Verification items for the finished model (mm, model axes). Face numbers are marked on the shaded views. A direction names the side the tool comes from. Give positions to 0.01 mm unless a question says otherwise; leave off trailing zeros. Order: outer loops, then holes, each group sorted by start corner. A loop starts at its lowest first (then second) coordinate and runs counter-clockwise, first axis right, second up. Notation, with made-up numbers: (-29.75, 45.5) - (-5.75, 45.5) arc R27 cw to (-5.75, 71.5) - close; hole circle Ø10 at (82, 2.5). An arc over 180 degrees is marked (long way). Answer as a JSON object with one key per item and string values. Group by question number.
(1) Access from +Z, -Z, +X, -X, +Y, -Y to the whole of each face (thin tool, end or side, straight path). Record for the marked faces 5, 6 and 7.
(2) Mould release check, pull along Z, two halves, no side actions. Record for the marked faces 1, 2, 3 and 4: +Z half, -Z half, draft (parallel to the pull), parting line (faces both ways), or undercut.
(3) Section check D-D (x = -7.5). Record the boundary of the cut face in (y, z), then the cut area to 3 significant figures.
(4) Thickness scan on line 1 (Y direction, x = -18, z = 0); line 2 (Y direction, x = -12.5, z = -0.25); line 3 (Z direction, x = -10.75, y = 5.25). Record the ranges inside material, lowest first.
(5) Section check B-B (x = -16.25). Record the boundary of the cut face in (y, z).
(6) Depth check by flat-ended pin: pin 1 Ø1 at (x, y) = (-4, 4.5) entering from -Z; pin 2 Ø4 at (x, z) = (-10.5, 9) entering from +Y; pin 3 Ø1 at (x, y) = (-18.5, -6) entering from +Z; pin 4 Ø1.1 at (y, z) = (8, 0) entering from -X. Enter the tip coordinate at first touch or a pass-through.
(7) Section check A-A (z = 0). Record the boundary of the cut face in (x, y).
(8) Section check C-C (y = 0). Record the boundary of the cut face in (x, z).
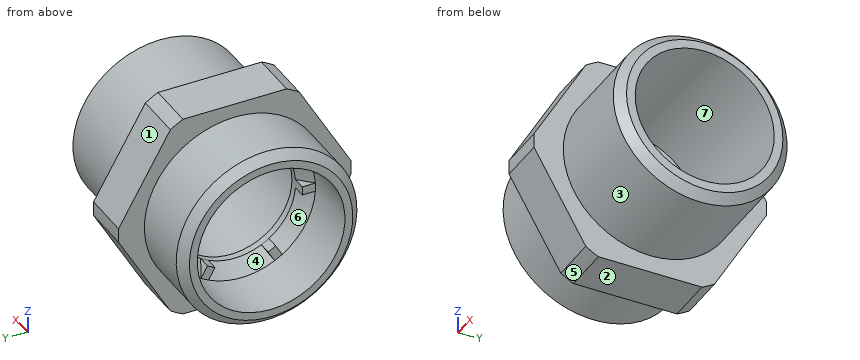
```python
from build123d import *

# Parameters (mm, degrees)
SKETCH_2_R               = 10
EXTRUDE_1_DEPTH          = 12
SKETCH_3_R               = 10
EXTRUDE_2_DEPTH          = 5.5
SKETCH_4_R               = 10.4
EXTRUDE_3_DEPTH          = 8
SKETCH_6_R               = 13.856406461
SKETCH_6_R_2             = 13.4
CUT_EXTRUDE_1_DEPTH      = 26.342651795
CHAMFER_1_SIZE           = 1
EXTRUDE_4_REACH          = 26.545
SKETCH_7_W               = 1
SKETCH_7_H               = 8.5
SKETCH_8_R               = 7
CUT_EXTRUDE_2_DEPTH      = 32.205928924
SKETCH_9_R               = 8.5
CUT_EXTRUDE_3_DEPTH      = 6.5
PATTERN_CIRCULAR_1_COUNT = 6


with BuildPart() as part:
    # Эскиз2 → Вытянуть1 (new body)
    with BuildSketch(Plane(origin=(0, 0, 0), x_dir=(0, 0, -1), z_dir=(1, 0, 0))):
        Circle(SKETCH_2_R)
    extrude(amount=-EXTRUDE_1_DEPTH)

    # Эскиз3 → Вытянуть2 (add)
    # profile 1 of 2: a face of its own
    with BuildSketch(Plane.ZY.offset(12)):
        Polygon((12, -6.92820323), (12, 6.92820323), (0, 13.856406461), (-12, 6.92820323), (-12, -6.92820323), (0, -13.856406461), align=None)
        with Locations(Location((0, 0, 0), (0, 0, 180))):
            Circle(SKETCH_3_R, mode=Mode.SUBTRACT)
    # profile 2 of 2: a face of its own
    with BuildSketch(Plane.ZY.offset(12)):
        with Locations(Location((0, 0, 0), (0, 0, 180))):
            Circle(SKETCH_3_R)
    extrude(amount=EXTRUDE_2_DEPTH)

    # Эскиз4 → Вытянуть3 (add)
    with BuildSketch(Plane.ZY.offset(17.5)):
        Circle(SKETCH_4_R)
    extrude(amount=EXTRUDE_3_DEPTH)

    # Эскиз5 → Вырез-Повернуть1 (revolve, cut)
    with BuildSketch(Plane.XY, mode=Mode.PRIVATE) as cut_revolve_1_sk:
        Polygon((0, 0), (0, 8), (-16.7, 8), (-16.7, 7), (-17.5, 7), (-19, 8.5), (-25.5, 8.5), (-25.5, 0), align=None)
    revolve(cut_revolve_1_sk.sketch.rotate(Axis((-25.5, 0, 0), (1, 0, 0)), 90), axis=Axis((-25.5, 0, 0), (1, 0, 0)), mode=Mode.SUBTRACT)

    # Эскиз6 → Вырез-Вытянуть1 (cut, through all)
    with BuildSketch(Plane.ZY.offset(17.5)):
        Circle(SKETCH_6_R)
        Circle(SKETCH_6_R_2, mode=Mode.SUBTRACT)
    extrude(amount=-CUT_EXTRUDE_1_DEPTH, mode=Mode.SUBTRACT)

    # Фаска1
    chamfer_1_edges = [part.edges().sort_by_distance(p)[0] for p in [
        (0, 0, 10),
        (-25.5, 0, -10.4),
    ]]
    chamfer(chamfer_1_edges, length=CHAMFER_1_SIZE)

    # Вытянуть4: up to this face of the body (flat: up to its plane)
    extrude_4_end = Plane(part.part.faces().sort_by_distance((-25.5, 0, -9.13412785))[0])
    # Эскиз7 → Вытянуть4 (add, up to the picked face)
    with BuildSketch(Plane(origin=(-16.7, 0, 0), x_dir=(0, 0, -1), z_dir=(1, 0, 0)), mode=Mode.PRIVATE) as extrude_4_sk1:
        with Locations((0, 4.25)):
            Rectangle(SKETCH_7_W, SKETCH_7_H)
    extrude_4_tool1 = split(extrude(extrude_4_sk1.sketch, amount=-EXTRUDE_4_REACH, mode=Mode.PRIVATE), bisect_by=extrude_4_end, keep=Keep.BOTH, mode=Mode.PRIVATE)
    add(extrude_4_tool1.solids().sort_by(Axis((-16.7, 4.25, 0), (-1, 0, 0)))[0])

    # Эскиз8 → Вырез-Вытянуть2 (cut, through all)
    with BuildSketch(Plane.ZY.offset(25.5)):
        Circle(SKETCH_8_R)
    extrude(amount=-CUT_EXTRUDE_2_DEPTH, mode=Mode.SUBTRACT)

    # Эскиз9 → Вырез-Вытянуть3 (cut)
    with BuildSketch(Plane.ZY.offset(25.5)):
        Circle(SKETCH_9_R)
    extrude(amount=-CUT_EXTRUDE_3_DEPTH, mode=Mode.SUBTRACT)

    # Круговой массив1: part ×6 about axis
    pattern_circular_1_axis = Axis((0, 0, 0), (1, 0, 0))


with BuildPart() as part_1:
    add(part.part)
    for i in range(1, PATTERN_CIRCULAR_1_COUNT):
        add(part.part.rotate(pattern_circular_1_axis, i * 360 / PATTERN_CIRCULAR_1_COUNT))


solid = part_1.part
```
Solutions:
{
 "1": {"face 5": "-Z, +X, -X, -Y", "face 6": "-X", "face 7": "+X"},
 "2": {"face 1": "+Z half", "face 2": "-Z half", "face 3": "parting line", "face 4": "undercut"},
 "3": {"outline": "circle Ø20 at (0, 0); hole circle Ø16 at (0, 0)", "area": "113 mm2"},
 "4": {"line 1": "y = -10.4 to -7, 7 to 10.4", "line 2": "y = -13.4 to -8, 8 to 13.4", "line 3": "z = -8.51 to -6.04, 6.04 to 8.51"},
 "5": {"outline": "(-13.37, -0.84) - (-7.41, -11.16) arc R13.4 ccw to (-5.96, -12) - (5.96, -12) arc R13.4 ccw to (7.41, -11.16) - (13.37, -0.84) arc R13.4 ccw to (13.37, 0.84) - (7.41, 11.16) arc R13.4 ccw to (5.96, 12) - (-5.96, 12) arc R13.4 ccw to (-7.41, 11.16) - (-13.37, 0.84) arc R13.4 ccw to start; hole circle Ø16 at (0, 0)"},
 "6": {"pin 1": "stops at z = -9.17", "pin 2": "stops at y = 9.42", "pin 3": "stops at z = 8.83", "pin 4": "stops at x = -25.5"},
 "7": {"outline": "(-25.5, -9.4) - (-24.5, -10.4) - (-17.5, -10.4) - (-17.5, -13.4) - (-12, -13.4) - (-12, -10) - (-1, -10) - (0, -9) - (0, -8) - (-16.7, -8) - (-16.7, -7) - (-19, -7) - (-19, -8.5) - (-25.5, -8.5) - close; (-25.5, 8.5) - (-19, 8.5) - (-19, 7) - (-16.7, 7) - (-16.7, 8) - (0, 8) - (0, 9) - (-1, 10) - (-12, 10) - (-12, 13.4) - (-17.5, 13.4) - (-17.5, 10.4) - (-24.5, 10.4) - (-25.5, 9.4) - close"},
 "8": {"outline": "(-25.5, -9.4) - (-24.5, -10.4) - (-17.5, -10.4) - (-17.5, -12) - (-12, -12) - (-12, -10) - (-1, -10) - (0, -9) - (0, -8) - (-16.7, -8) - (-16.7, -7) - (-17.5, -7) - (-19, -8.5) - (-25.5, -8.5) - close; (-25.5, 8.5) - (-19, 8.5) - (-17.5, 7) - (-16.7, 7) - (-16.7, 8) - (0, 8) - (0, 9) - (-1, 10) - (-12, 10) - (-12, 12) - (-17.5, 12) - (-17.5, 10.4) - (-24.5, 10.4) - (-25.5, 9.4) - close"}
}
